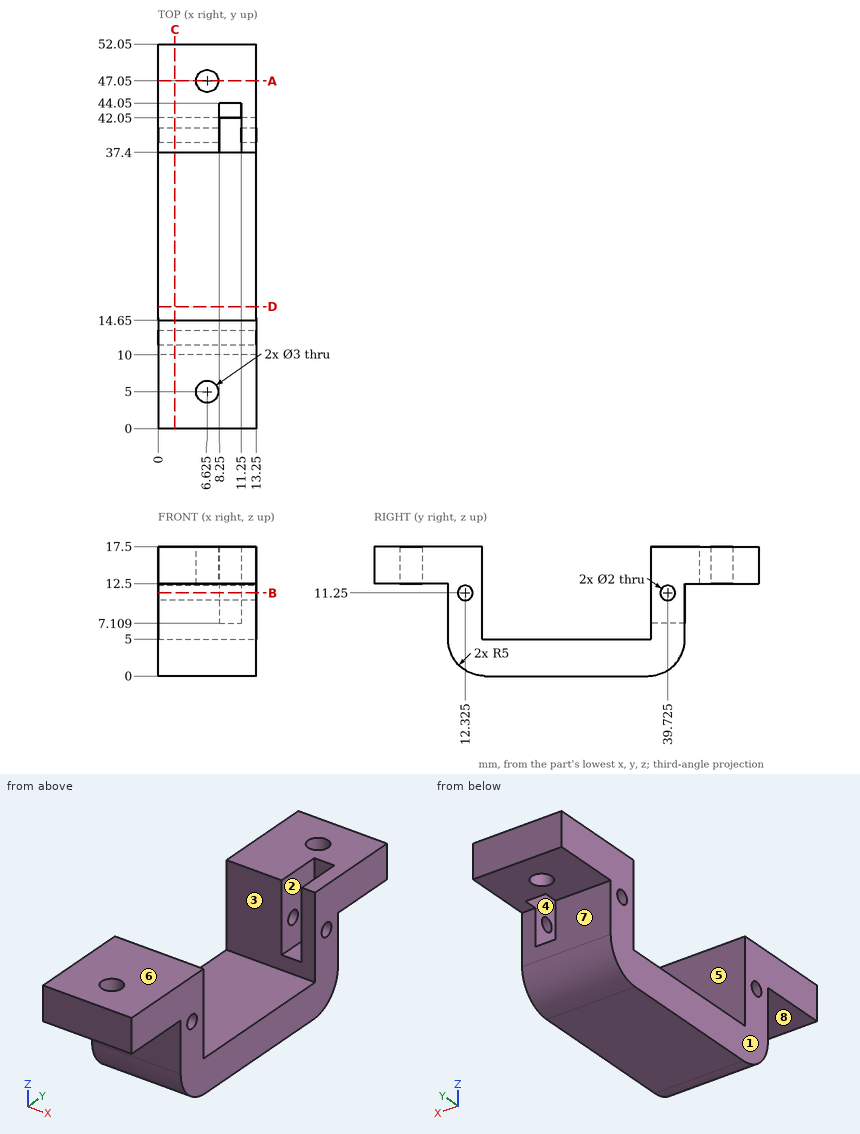
Here's the drawing with two shaded views (mm, measured from the low corner). I have some questions. A direction names the side the tool comes from. Give positions to 0.01 mm unless a question says otherwise; leave off trailing zeros. Loops run counter-clockwise (first coordinate to the right, second up) from the corner with the lowest first, then second, coordinate; pieces in that order, holes last. Notation, with made-up numbers: (24.5, -21) - (58.5, -21) arc R9 ccw to (58.5, -17) - close; hole circle Ø8 at (11.25, 14). An arc over 180 degrees is marked (long way). One line per item, written item: value.
(1) I need wall thicknesses on line 1 along Y through (x, z) = (3.5, 11.25) (3 decimals); line 2 along Y through (x, z) = (12, 7); line 3 along Y through (x, z) = (4.5, 13.75). Which ranges of each line are inside material? Lowest first, please.
Verdict:
line 1: 10 to 11.325, 13.325 to 14.65, 37.4 to 38.725, 40.725 to 42.05
line 2: 10 to 14.65, 37.4 to 42.05
line 3: 0 to 14.65, 37.4 to 52.05
(2) If we section it at A-A, the plane y = 47.05: List the corners of the cut face in (x, z) for me (3 decimals), plus the area to 4 significant figures.
Verdict:
outline: (0, 12.5) - (5.125, 12.5) - (5.125, 17.5) - (0, 17.5) - close; (8.125, 12.5) - (13.25, 12.5) - (13.25, 17.5) - (8.125, 17.5) - close
area: 51.25 mm^2
(3) On a 3-axis mill with a long thin cutter (end or side, diameter ignored), from which of +Z, -Z, +X, -X, +Y, -Y can I reach the whole of each face in a straight line? I mean the marked faces 4, 5, 6, 7 and 8. Say none if no direction works.
Verdict:
face 4: +Z
face 5: +Z, +X, -X
face 6: +Z, +X, -X, +Y, -Y
face 7: -Z, +X, -X, +Y
face 8: -Z, +X, -X, -Y
(4) If we section it at D-D, the plane y = 16.5: List the corners of the cut face in (x, z) for me, plus the area to 4 significant figures.
Verdict:
outline: (0, 0) - (13.25, 0) - (13.25, 5) - (0, 5) - close
area: 66.25 mm^2
(5) If we mould it in two halves opening along X, with no side actions, what happens to the marked faces 1, 2 and 3? For each: released by +X, released by -X, zero draft, split by the parting line, or undercut.
Verdict:
face 1: released by -X
face 2: undercut
face 3: zero draft
(6) If we section it at C-C, the plane x = 2.25: List the corners of the cut face in (y, z) for me (3 decimals), plus the area to 3 significant figures.
Verdict:
outline: (0, 12.5) - (10, 12.5) - (10, 5) arc R5 ccw to (15, 0) - (37.05, 0) arc R5 ccw to (42.05, 5) - (42.05, 12.5) - (52.05, 12.5) - (52.05, 17.5) - (37.4, 17.5) - (37.4, 5) - (14.65, 5) - (14.65, 17.5) - (0, 17.5) - close; hole circle Ø2 at (12.325, 11.25); hole circle Ø2 at (39.725, 11.25)
area: 359 mm^2
(7) If we section it at B-B, the plane z = 11.25: List the corners of the cut face in (x, y) for me (3 decimals), plus the area to 3 significant figures.
Verdict:
outline: (0, 10) - (13.25, 10) - (13.25, 11.325) - (0, 11.325) - close; (0, 13.325) - (13.25, 13.325) - (13.25, 14.65) - (0, 14.65) - close; (0, 37.4) - (8.25, 37.4) - (8.25, 38.725) - (0, 38.725) - close; (0, 40.725) - (8.25, 40.725) - (8.25, 42.05) - (0, 42.05) - close; (11.25, 37.4) - (13.25, 37.4) - (13.25, 38.725) - (11.25, 38.725) - close; (11.25, 40.725) - (13.25, 40.725) - (13.25, 42.05) - (11.25, 42.05) - close
area: 62.3 mm^2
(8) I'm going to push flat-ended pins straight in: pin 1 (2 mm diameter, centred on x = 9, z = 7.5, fed in from -Y); pin 2 (1 mm diameter, centred on x = 6.5, z = 4, fed in from +Y); pin 3 (6.5 mm diameter, centred on x = 4, y = 26.5, fed in from +Z); pin 4 (1.2 mm diameter, centred on y = 12.325, z = 11.25, fed in from -X). Where does each tip first touch, or does it pass through?
Verdict:
pin 1: y = 10
pin 2: y = 42.02
pin 3: z = 5
pin 4: through
